```python
from build123d import *

# Parameters (mm, degrees)
SKETCH_1_R           = 23
EXTRUDE_1_DEPTH      = 30
CUT_EXTRUDE_1_DEPTH  = 50
SKETCH_10_R          = 12.5
CUT_EXTRUDE_6_DEPTH  = 426.323406363
SKETCH_15_R          = 5
CUT_EXTRUDE_8_DEPTH  = 426.323406363
SKETCH_16_W          = 600
SKETCH_16_H          = 120
EXTRUDE_2_DEPTH      = 30
CUT_EXTRUDE_9_REACH  = 427.323
SKETCH_17_R          = 26
EXTRUDE_START        = -5
SKETCH_18_R          = 26
EXTRUDE_3_DEPTH      = 5
SKETCH_19_R          = 6
CUT_EXTRUDE_10_DEPTH = 58


with BuildPart() as part:
    # 草图1 → 凸台-拉伸1 (new body)
    with BuildSketch(Plane.XY):
        with BuildLine():
            Line((0, 0), (-295.442325904, -52.0944533))
            ThreePointArc((-295.442325904, -52.0944533), (0, 300), (295.442325904, -52.0944533))
            Line((295.442325904, -52.0944533), (0, 0))
        make_face()
        with Locations((-125, 216.506350946)):
            Circle(SKETCH_1_R, mode=Mode.SUBTRACT)
        with Locations((-216.506350946, 125)):
            Circle(SKETCH_1_R, mode=Mode.SUBTRACT)
        with Locations((216.506350946, 125)):
            Circle(SKETCH_1_R, mode=Mode.SUBTRACT)
        with Locations((125, 216.506350946)):
            Circle(SKETCH_1_R, mode=Mode.SUBTRACT)
    extrude(amount=EXTRUDE_1_DEPTH)

    # 草图2 → 切除-拉伸1 (cut)
    with BuildSketch(Plane.XY.offset(30)):
        with BuildLine():
            Line((0, 0), (-250, 0))
            ThreePointArc((-250, 0), (0, -250), (250, 0))
            Line((250, 0), (0, 0))
        make_face()
    extrude(amount=-CUT_EXTRUDE_1_DEPTH, mode=Mode.SUBTRACT)

    # 草图10 → 切除-拉伸6 (cut, through all)
    with BuildSketch(Plane.XY.offset(30)):
        with Locations((-246.201938253, 43.412044417)):
            Circle(SKETCH_10_R)
        with Locations(Location((246.201938253, 43.412044417, 0), (0, 0, 180))):
            Circle(SKETCH_10_R)
        with Locations((-64.704761276, 241.481456572)):
            Circle(SKETCH_10_R)
        with Locations(Location((64.704761276, 241.481456572, 0), (0, 0, 180))):
            Circle(SKETCH_10_R)
    extrude(amount=-CUT_EXTRUDE_6_DEPTH, mode=Mode.SUBTRACT)

    # 草图15 → 切除-拉伸8 (cut, through all)
    with BuildSketch(Plane.XY.offset(30)):
        with Locations((-257.081286775, 104.872747053)):
            Circle(SKETCH_15_R)
        with Locations((-105.443118667, 246.486099918)):
            Circle(SKETCH_15_R)
        with Locations((-27.326692423, 54.2718973)):
            Circle(SKETCH_15_R)
        with Locations(Location((27.326692423, 54.2718973, 0), (0, 0, 180))):
            Circle(SKETCH_15_R)
        with Locations(Location((105.443118667, 246.486099918, 0), (0, 0, 180))):
            Circle(SKETCH_15_R)
        with Locations(Location((257.081286775, 104.872747053, 0), (0, 0, 180))):
            Circle(SKETCH_15_R)
    extrude(amount=-CUT_EXTRUDE_8_DEPTH, mode=Mode.SUBTRACT)

    # 草图16 → 凸台-拉伸2 (add)
    with BuildSketch(Plane.XY.offset(30)):
        with Locations((0, -60)):
            Rectangle(SKETCH_16_W, SKETCH_16_H)
    extrude(amount=-EXTRUDE_2_DEPTH)

    # 草图17 → 切除-拉伸9 (cut, up to next)
    with BuildSketch(Plane.XY.offset(30), mode=Mode.PRIVATE) as cut_extrude_9_sk1:
        with Locations((-120.47, 120.47)):
            Circle(SKETCH_17_R)
    cut_extrude_9_tool1 = extrude(cut_extrude_9_sk1.sketch, amount=-CUT_EXTRUDE_9_REACH, mode=Mode.PRIVATE) & part.part
    # 草图17 → 切除-拉伸9 (cut, up to next)
    with BuildSketch(Plane.XY.offset(30), mode=Mode.PRIVATE) as cut_extrude_9_sk2:
        with Locations((120.47, 120.47)):
            Circle(SKETCH_17_R)
    cut_extrude_9_tool2 = extrude(cut_extrude_9_sk2.sketch, amount=-CUT_EXTRUDE_9_REACH, mode=Mode.PRIVATE) & part.part
    add(cut_extrude_9_tool1.solids().sort_by_distance((-120.47, 120.47, 30))[0], mode=Mode.SUBTRACT)
    add(cut_extrude_9_tool2.solids().sort_by_distance((120.47, 120.47, 30))[0], mode=Mode.SUBTRACT)

    # 草图18 → 凸台-拉伸3 (add)
    with BuildSketch(Plane(origin=(0, 0, 0), x_dir=(-1, 0, 0), z_dir=(0, 0, -1)).offset(EXTRUDE_START)):
        with Locations(Location((120.47, 120.47, 0), (0, 0, 180))):
            Circle(SKETCH_18_R)
        with Locations((-120.47, 120.47)):
            Circle(SKETCH_18_R)
    extrude(amount=EXTRUDE_3_DEPTH)

    # 草图19 → 切除-拉伸10 (cut)
    with BuildSketch(Plane(origin=(0, 0, 0), x_dir=(-1, 0, 0), z_dir=(0, 0, -1))):
        with Locations((0, 80)):
            Circle(SKETCH_19_R)
    extrude(amount=-CUT_EXTRUDE_10_DEPTH, mode=Mode.SUBTRACT)


solid = part.part
```
The listing builds one solid part. Answer for the finished solid, in the listing's coordinates (mm). A direction names the side the tool comes from. Round coordinates to 2 decimals unless told otherwise and drop trailing zeros. Loops run counter-clockwise (first coordinate to the right, second up) from the corner with the lowest first, then second, coordinate; pieces in that order, holes last.
1) A cutting plane is placed at A-A on x = 0. Determine the outline of the cut face in (y, z), plus the area to 3 significant figures.
Outcome:
outline: (-120, 0) - (74, 0) - (74, 30) - (-120, 30) - close; (86, 0) - (300, 0) - (300, 30) - (86, 30) - close
area: 12,200 mm2
2) For faces 5 (the face through (-234.655, 38.624, 15.21)), 6 (the face through (145.27, 128.28, 17.68)), determine the directions among +Z, -Z, +X, -X, +Y, -Y from which every point of the face is accessible in a straight line to the end or side of a thin tool.
Outcome:
face 5: +Z, -Z
face 6: +Z
3) Given P1, Ø1, axis at y = 178.5, z = 13.5, coming from the +X side; P2, Ø15.5, axis at x = -121, y = 120, coming from the +Z side; P3, Ø2, axis at y = 249.5, z = 10, coming from the +X side; P4, Ø14, axis at x = 0, y = 80, coming from the -Z side, each flat-ended and moving along its own axis, determine where each tip first touches the part or whether it passes through.
Outcome:
P1: stops at x = 241.49
P2: stops at z = 5
P3: stops at x = 168.07
P4: stops at z = 0
4) For a pull along X with two mould halves and no side action, classify faces 1 (the face through (58.937, 252.571, 15.21)), 2 (the face through (-95.67, 128.28, 17.68)), 3 (the face through (300, -61, 15)), 4 (the face through (-300, -61, 15)) as released by +X, released by -X, zero draft, split by the parting line, or undercut.
Outcome:
face 1: undercut
face 2: undercut
face 3: released by +X
face 4: released by -X
5) A cutting plane is placed at C-C on y = 133.5. Determine the outline of the cut face in (x, z), plus the area to 3 significant figures.
Outcome:
outline: (-268.66, 0) - (-237.88, 0) - (-237.88, 30) - (-268.66, 30) - close; (-195.13, 0) - (195.13, 0) - (195.13, 30) - (142.97, 30) - (142.97, 5) - (97.97, 5) - (97.97, 30) - (-97.97, 30) - (-97.97, 5) - (-142.97, 5) - (-142.97, 30) - (-195.13, 30) - close; (237.88, 0) - (268.66, 0) - (268.66, 30) - (237.88, 30) - close
area: 11,300 mm2
6) Consider line 1 (X direction, y = 120.47, z = 13.5); line 2 (Y direction, x = -120.47, z = 13.25); line 3 (X direction, y = 227, z = 18). Determine where each line is inside the solid, lowest interval first.
Outcome:
line 1: x = -274.75 to -239.06, -193.96 to -146.47, -94.47 to 94.47, 146.47 to 193.96, 239.06 to 274.75
line 2: y = -120 to 94.47, 146.47 to 193.96, 239.06 to 274.75
line 3: x = -196.14 to -145.47, -104.53 to 104.53, 145.47 to 196.14
7) A cutting plane is placed at D-D on y = 80. Determine the outline of the cut face in (x, z).
Outcome:
outline: (-289.14, 0) - (-6, 0) - (-6, 30) - (-289.14, 30) - close; (6, 0) - (289.14, 0) - (289.14, 30) - (6, 30) - close
8) A cutting plane is placed at B-B on z = 9.5. Give the number of separate pieces and of enclosed holes in the cut face, plus the area to 3 significant figures.
Outcome:
separate pieces: 1
enclosed holes: 17
area: 200,000 mm2
